from build123d import *

# Parameters (mm, degrees)
F1_DEPTH  = 19
F2_R      = 3
F3_DEPTH  = 3
F4_R      = 1.5
F5_DEPTH  = 7.5
F6_R      = 1.05
F7_DEPTH  = 1
F8_R      = 16.5
F9_DEPTH  = 5
F10_W     = 10
F10_H     = 6
F11_DEPTH = 5


# Not quite as in the source:
# - a pattern or mirror of a feature is missing from the dataset's text; its kind, count and spacing are read off the source's solid


with BuildPart() as f1:
    # F0 (on Front) → F1 (new body)
    with BuildSketch(Plane.XZ):
        with BuildLine():
            Line((7.3, -17), (7.3, -11.9461290802))
            ThreePointArc((7.3, -11.9461290802), (0, 14), (-7.3, -11.9461290802))
            Line((-7.3, -11.9461290802), (-7.3, -17))
            Line((-7.3, -17), (7.3, -17))
        make_face()
    extrude(amount=F1_DEPTH)

    # F2 (on face) → F3 (join)
    with BuildSketch(Plane.XZ.offset(19)):
        with Locations((0, 8)):
            Circle(F2_R)
    extrude(amount=F3_DEPTH)

    # F4 (on face) → F5 (join)
    with BuildSketch(Plane.XZ.offset(22)):
        with Locations((0, 8)):
            Circle(F4_R)
    extrude(amount=F5_DEPTH)

    # F6 (on face) → F7 (join)
    with BuildSketch(Plane.XZ.offset(19)):
        with BuildLine():
            Line((13.8901943831, -1.75), (17.5, -1.75))
            ThreePointArc((17.5, -1.75), (19.25, 0), (17.5, 1.75))
            Line((17.5, 1.75), (13.8901943831, 1.75))
            Line((13.8901943831, 1.75), (13.8901943831, -1.75))
        make_face()
        with Locations((17.5, 0)):
            Circle(F6_R, mode=Mode.SUBTRACT)
    f7 = extrude(amount=-F7_DEPTH)

    # F7_copies: F7 across plane
    add(f7.mirror(Plane(origin=(0, 0, 0), x_dir=(0, 0, -1), z_dir=(-1, 0, 0))))

    # F8 (on face) → F9 (join)
    with BuildSketch(Plane.XZ.offset(22)):
        with Locations((0, 8)):
            Circle(F8_R)
    extrude(amount=F9_DEPTH)

    # F10 (on face) → F11 (join)
    with BuildSketch(Plane(origin=(0, 0, -17), x_dir=(1, 0, 0), z_dir=(0, 0, -1))):
        with Locations((0, 14)):
            Rectangle(F10_W, F10_H)
    extrude(amount=F11_DEPTH)


solid = f1.part
Part model, mm, in its own coordinate system. A direction names the side the tool comes from. Give positions to 0.01 mm unless a question says otherwise; leave off trailing zeros. Write each loop counter-clockwise with the first axis right and the second up, starting at its lowest first coordinate (ties: lowest second). Pieces come first, ordered by that corner, then holes.
1) Cut at A-A on x = 0. Write the cut outline in (y, z), then the cut area to 4 significant figures.
Resolved:
outline: (-29.5, 6.5) - (-27, 6.5) - (-27, -8.5) - (-22, -8.5) - (-22, 5) - (-19, 5) - (-19, -17) - (-17, -17) - (-17, -22) - (-11, -22) - (-11, -17) - (0, -17) - (0, 14) - (-19, 14) - (-19, 11) - (-22, 11) - (-22, 24.5) - (-27, 24.5) - (-27, 9.5) - (-29.5, 9.5) - close
area: 809.5 mm2
2) Pin check, flat tips, straight feed: pin 1 (4 mm diameter, centred on y = -15, z = -19.5, fed in from +X); pin 2 (10 mm diameter, centred on x = -15, y = -16.5, fed in from -Z); pin 3 (2 mm diameter, centred on x = 4.5, z = -8.5, fed in from -Y). Stop position of each tip, or through.
Resolved:
pin 1: stops at x = 5
pin 2: stops at z = -9.8
pin 3: stops at y = -27
3) Cut at C-C on z = 0. Write the cut outline in (x, y), then the cut area to 3 significant figures.
Resolved:
outline: (-19.25, -19) - (-18.55, -19) - (-18.55, -18) - (-19.25, -18) - close; (-16.45, -19) - (16.45, -19) - (16.45, -18) - (14, -18) - (14, 0) - (-14, 0) - (-14, -18) - (-16.45, -18) - close; (-14.43, -27) - (14.43, -27) - (14.43, -22) - (-14.43, -22) - close; (18.55, -19) - (19.25, -19) - (19.25, -18) - (18.55, -18) - close
area: 683 mm2
4) Two-plate mould, pull along Y, no slides. Class faces 1 (the face through (-0.2, -22, 4.6)), 2 (the face through (0, -17, -19)), 3 (the face through (-0.325, -28.232, 6.536)), 4 (the face through (0, -19, -1)): released by +Y, released by -Y, zero draft, split by the parting line, or undercut.
Resolved:
face 1: undercut
face 2: released by -Y
face 3: zero draft
face 4: undercut
5) Which spindle directions (+Z, -Z, +X, -X, +Y, -Y) get a long thin tool onto all of the face, cutting with end or side? Do faces 5 (the face through (0.51, -9.37, 13.99)), 6 (the face through (7.3, -9, -15)), 7 (the face through (8.87, -24.465, 21.913)). Say none if no direction does.
Resolved:
face 5: +Y
face 6: -Z, +X, +Y, -Y
face 7: -Y
6) Cut at B-B on x = 12. Write the cut outline in (y, z).
Resolved:
outline: (-27, -3.32) - (-22, -3.32) - (-22, 19.32) - (-27, 19.32) - close; (-19, -7.21) - (0, -7.21) - (0, 7.21) - (-19, 7.21) - close
7) Probe L1, parallel to Z at x = -17.5, y = -18.8; L2, parallel to Y at x = -1, z = -1.5. List the from-to ranges inside material, lowest first.
Resolved:
L1: z = -1.75 to -1.05, 1.05 to 1.75
L2: y = -27 to -22, -19 to 0
8) Cut at D-D on y = -26.25. Write the cut outline in (x, z), then the cut area to 3 significant figures.
Resolved:
outline: circle Ø33 at (0, 8)
area: 855 mm2
